Work out the finished part from the listing and answer in its coordinate system (mm). A direction names the side the tool comes from. Coordinates: 2 decimals unless noted, no trailing zeros. Order: outer loops, then holes, each group sorted by start corner. A loop starts at its lowest first (then second) coordinate and runs counter-clockwise, first axis right, second up. Notation, with made-up numbers: (34, 51) -> (64, 51) arc R18 cw to (64, 78) -> close; hole circle Ø5 at (68.5, 19). An arc over 180 degrees is marked (long way). Use one line per item in the form item = value.
from build123d import *

# Parameters (mm, degrees)
F0_R     = 4.7625
F0_W     = 3.175
F0_H     = 25.4
F1_DEPTH = 3.175


with BuildPart() as f1:
    # F0 (on Top) → F1 (new body)
    with BuildSketch(Plane.XY):
        Polygon((25.4, 12.7), (25.4, 25.4), (12.7, 25.4), (12.7, 22.225), (-12.7, 22.225), (-12.7, 25.4), (-25.4, 25.4), (-25.4, 12.7), (-22.225, 12.7), (-22.225, -12.7), (-25.4, -12.7), (-25.4, -25.4), (-12.7, -25.4), (-12.7, -22.225), (12.7, -22.225), (12.7, -25.4), (25.4, -25.4), (25.4, -12.7), (22.225, -12.7), (22.225, 12.7), align=None)
        Circle(F0_R, mode=Mode.SUBTRACT)
        with Locations((-26.9875, 0)):
            Rectangle(F0_W, F0_H)
        with Locations((-23.8125, 0)):
            Rectangle(F0_W, F0_H)
        with Locations((26.9875, 0)):
            Rectangle(F0_W, F0_H)
        with Locations((23.8125, 0)):
            Rectangle(F0_W, F0_H)
    extrude(amount=F1_DEPTH)


solid = f1.part
(1) Straight lines are drawn through the part: line 1 along Y through (x, z) = (0, 2.3) (1 decimal); line 2 along Y through (x, z) = (2, 2.1) (3 decimals); line 3 along Y through (x, z) = (8, 2.35) (3 decimals). For each, find the intervals that lie inside material, in ascending order.
Data:
line_1 = -22.2 to -4.8, 4.8 to 22.2
line_2 = -22.225 to -4.322, 4.322 to 22.225
line_3 = -22.225 to 22.225
(2) Section A-A on x = 0 is taken. Write down the section's boundary in (y, z) (1 decimal), plus the area to 3 significant figures.
Data:
outline = (-22.2, 0) -> (-4.8, 0) -> (-4.8, 3.2) -> (-22.2, 3.2) -> close; (4.8, 0) -> (22.2, 0) -> (22.2, 3.2) -> (4.8, 3.2) -> close
area = 111 mm²
(3) Section D-D on x = 8.5 is taken. Write down the section's boundary in (y, z) (3 decimals).
Data:
outline = (-22.225, 0) -> (22.225, 0) -> (22.225, 3.175) -> (-22.225, 3.175) -> close
(4) Which of the six approach directions +Z, -Z, +X, -X, +Y, -Y give full straight-line access (tool end or side, diameter ignored) to faces 1 (the flat face through (27, -12.7, 2)), 2 (the flat face through (-25.4, -19, 2)), 3 (the flat face through (27, 12.7, 2)), 4 (the flat face through (-12.7, -24, 2))?
Data:
face_1 = +Z, -Z, +X, -Y
face_2 = +Z, -Z, -X, -Y
face_3 = +Z, -Z, +X, +Y
face_4 = +Z, -Z, -Y
(5) The mould has two halves that part along X. Classify faces 5 (the flat face through (19, 25.4, 2)), 6 (the flat face through (12.7, -24, 2)), 7 (the flat face through (-25.4, 19, 2)): released by +X, released by -X, zero draft, split by the parting line, or undercut.
Data:
face_5 = zero draft
face_6 = undercut
face_7 = released by -X
(6) Each of these flat-tipped pins is pushed along its axis until it touches: P1, Ø1, axis at x = -27.5, z = 1.5, coming from the +Y side; P2, Ø1, axis at x = 1, z = 0.5, coming from the +Y side (3 decimals); P3, Ø1, axis at y = 18.5, z = 2, coming from the +X side. Where does it stop, or does it pass through?
Data:
P1 = 12.7
P2 = 22.225
P3 = 25.4
(7) Section C-C on z = 1.45 is taken. Write down the section's boundary in (x, y) (1 decimal), plus the area to 3 significant figures.
Data:
outline = (-28.6, -12.7) -> (-25.4, -12.7) -> (-25.4, -25.4) -> (-12.7, -25.4) -> (-12.7, -22.2) -> (12.7, -22.2) -> (12.7, -25.4) -> (25.4, -25.4) -> (25.4, -12.7) -> (28.6, -12.7) -> (28.6, 12.7) -> (25.4, 12.7) -> (25.4, 25.4) -> (12.7, 25.4) -> (12.7, 22.2) -> (-12.7, 22.2) -> (-12.7, 25.4) -> (-25.4, 25.4) -> (-25.4, 12.7) -> (-28.6, 12.7) -> close; hole circle Ø9.5 at (0, 0)
area = 2,510 mm²
(8) Section B-B on y = 0 is taken. Write down the section's boundary in (x, z) (1 decimal), plus the area to 3 significant figures.
Data:
outline = (-28.6, 0) -> (-4.8, 0) -> (-4.8, 3.2) -> (-28.6, 3.2) -> close; (4.8, 0) -> (28.6, 0) -> (28.6, 3.2) -> (4.8, 3.2) -> close
area = 151 mm²
